from build123d import *

# Parameters (mm, degrees)
F1_DEPTH = 127


with BuildPart() as f1:
    # F0 (on Front) → F1 (new body)
    with BuildSketch(Plane.XZ):
        with BuildLine():
            Line((25.418775, -10.188777), (22.881775, -10.722313))
            ThreePointArc((22.881775, -10.722313), (21.269347, -11.748756), (20.039052, -13.211589))
            ThreePointArc((20.039052, -13.211589), (20.74222, -16.628007), (20.245645, -20.08051))
            ThreePointArc((20.245645, -20.08051), (21.413679, -21.348552), (22.881775, -22.252392))
            Line((22.881775, -22.252392), (25.418775, -22.785928))
            Line((25.418775, -22.785928), (27.955776, -22.252392))
            ThreePointArc((27.955776, -22.252392), (29.344167, -21.413137), (30.472134, -20.247089))
            ThreePointArc((30.472134, -20.247089), (29.994965, -16.699634), (30.798498, -13.211589))
            ThreePointArc((30.798498, -13.211589), (29.568203, -11.748756), (27.955776, -10.722313))
            Line((27.955776, -10.722313), (25.418775, -10.188777))
        make_face()
    extrude(amount=-F1_DEPTH)


solid = f1.part
Part model, mm, in its own coordinate system. Coordinates: 2 decimals unless noted, no trailing zeros. Order: outer loops, then holes, each group sorted by start corner. A loop starts at its lowest first (then second) coordinate and runs counter-clockwise, first axis right, second up. Notation, with made-up numbers: M 35.25,51.25 L 59.25,51.25 A33 cw 59.25,79.25 Z; hole C 1,16.25 d3. An arc over 180 degrees is marked long. One line per question, with ' | ' between items.
Q1. Slice it at B-B (z = -17). Give the cut face in (x, y), and give its area (3 significant figures).
A:
outline: M 20.75,0 L 29.99,0 L 29.99,127 L 20.75,127 Z | area: 1,170 mm^2
Q2. Slice it at C-C (x = 26.75). Give the cut face in (y, z).
A:
outline: M 0,-22.51 L 127,-22.51 L 127,-10.47 L 0,-10.47 Z
Q3. Two-plate mould, pull along Z, no slides. Class faces 1 (the face through (21, 63, -12)), 2 (the face through (29.993, 62.611, -16.75)), 3 (the face through (26.67, 62.611, -22.523)): +Z half, -Z half, draft (parallel to the pull), parting line (faces both ways), or undercut.
A:
face 1: +Z half | face 2: undercut | face 3: -Z half
Q4. Slice it at A-A (y = 75.5). Give the cut face in (x, z).
A:
outline: M 20.04,-13.21 A10.14 cw 20.25,-20.08 A6.3 ccw 22.88,-22.25 L 25.42,-22.79 L 27.96,-22.25 A6.3 ccw 30.47,-20.25 A9.99 cw 30.8,-13.21 A6.3 ccw 27.96,-10.72 L 25.42,-10.19 L 22.88,-10.72 A6.3 ccw Z
Q5. Drill centre lines: line 1 (X direction, y = 32, z = -16.5); line 2 (Z direction, x = 28, y = 26); line 3 (Z direction, x = 25.5, y = 43). Where is each one in solid material? Low to high.
A:
line 1: x = 20.74 to 30.01 | line 2: z = -22.23 to -10.74 | line 3: z = -22.77 to -10.21
Q6. Pin check, flat tips, straight feed: P1, Ø1.5, axis at x = 22.5, y = 80.5, coming from the -Z side; P2, Ø1, axis at x = 26, y = 83.5, coming from the -Z side; P3, Ø1.5, axis at x = 26.5, y = 89.5, coming from the -Z side. Stop position of each tip, or through.
A:
P1: stops at z = -22.33 | P2: stops at z = -22.77 | P3: stops at z = -22.72
